from build123d import *

# Parameters (mm, degrees)
SKETCH1_W           = 67.8
SKETCH1_H           = 11.732307158
SKETCH1_R           = 1.25
BOSS_EXTRUDE1_DEPTH = 3
SKETCH1_7_R         = 0.5
BOSS_EXTRUDE2_DEPTH = 2
FILLET1_R           = 6


with BuildPart() as part:
    # Sketch1 → Boss-Extrude1 (new body)
    with BuildSketch(Plane(origin=(0, 0, 0), x_dir=(1, 0, 0), z_dir=(0, 1, 0))):
        with Locations((8.337190195, 0)):
            Rectangle(SKETCH1_W, SKETCH1_H)
        with Locations(Location((-4.662809805, -3.5, 0), (0, 0, 270))):
            Circle(SKETCH1_R, mode=Mode.SUBTRACT)
        with BuildLine():
            ThreePointArc((-15.948035413, -2.8), (-22.562809805, 0), (-15.948035413, 2.8))
            Line((-15.948035413, 2.8), (-3.54760873, 2.1))
            ThreePointArc((-3.54760873, 2.1), (-1.562809805, 0), (-3.54760873, -2.1))
            Line((-3.54760873, -2.1), (-15.948035413, -2.8))
        make_face(mode=Mode.SUBTRACT)
        with Locations(Location((-4.662809805, 3.5, 0), (0, 0, 270))):
            Circle(SKETCH1_R, mode=Mode.SUBTRACT)
        with BuildLine():
            Line((32.622415803, -2.8), (20.221989119, -2.1))
            ThreePointArc((20.221989119, -2.1), (18.237190195, 0), (20.221989119, 2.1))
            Line((20.221989119, 2.1), (32.622415803, 2.8))
            ThreePointArc((32.622415803, 2.8), (36.85745002, 3.591491343), (39.237190195, 0))
            ThreePointArc((39.237190195, 0), (36.85745002, -3.591491343), (32.622415803, -2.8))
        make_face(mode=Mode.SUBTRACT)
    extrude(amount=BOSS_EXTRUDE1_DEPTH)

    # Sketch1<7> → Boss-Extrude2 (add)
    # profile 1 of 2: a face of its own
    with BuildSketch(Plane(origin=(0, 0, 0), x_dir=(1, 0, 0), z_dir=(0, 1, 0))):
        with BuildLine():
            Line((-3.54760873, 2.1), (-15.948035413, 2.8))
            ThreePointArc((-15.948035413, 2.8), (-15.071318463, 1.520259825), (-14.762809805, 0))
            ThreePointArc((-14.762809805, 0), (-15.071318463, -1.520259825), (-15.948035413, -2.8))
            Line((-15.948035413, -2.8), (-3.54760873, -2.1))
            ThreePointArc((-3.54760873, -2.1), (-1.562809805, 0), (-3.54760873, 2.1))
        make_face()
        with Locations(Location((-13.331400804, 0, 0), (0, 0, 270))):
            Circle(SKETCH1_7_R, mode=Mode.SUBTRACT)
        with Locations(Location((-11.331400804, 0, 0), (0, 0, 270))):
            Circle(SKETCH1_7_R, mode=Mode.SUBTRACT)
        with Locations(Location((-9.331400804, 0, 0), (0, 0, 270))):
            Circle(SKETCH1_7_R, mode=Mode.SUBTRACT)
        with Locations(Location((-7.331400804, 0, 0), (0, 0, 270))):
            Circle(SKETCH1_7_R, mode=Mode.SUBTRACT)
        with Locations(Location((-5.331400804, 0, 0), (0, 0, 270))):
            Circle(SKETCH1_7_R, mode=Mode.SUBTRACT)
        with Locations(Location((-3.331400804, 0, 0), (0, 0, 270))):
            Circle(SKETCH1_7_R, mode=Mode.SUBTRACT)
    # profile 2 of 2: a face of its own
    with BuildSketch(Plane(origin=(0, 0, 0), x_dir=(1, 0, 0), z_dir=(0, 1, 0))):
        with BuildLine():
            ThreePointArc((20.221989119, 2.1), (18.237190195, 0), (20.221989119, -2.1))
            Line((20.221989119, -2.1), (32.622415803, -2.8))
            ThreePointArc((32.622415803, -2.8), (31.437190195, 0), (32.622415803, 2.8))
            Line((32.622415803, 2.8), (20.221989119, 2.1))
        make_face()
        with Locations(Location((22.005781193, 0, 0), (0, 0, 270))):
            Circle(SKETCH1_7_R, mode=Mode.SUBTRACT)
        with Locations(Location((24.005781193, 0, 0), (0, 0, 270))):
            Circle(SKETCH1_7_R, mode=Mode.SUBTRACT)
        with Locations(Location((26.005781193, 0, 0), (0, 0, 270))):
            Circle(SKETCH1_7_R, mode=Mode.SUBTRACT)
        with Locations(Location((28.005781193, 0, 0), (0, 0, 270))):
            Circle(SKETCH1_7_R, mode=Mode.SUBTRACT)
        with Locations(Location((30.005781193, 0, 0), (0, 0, 270))):
            Circle(SKETCH1_7_R, mode=Mode.SUBTRACT)
        with Locations(Location((20.005781193, 0, 0), (0, 0, 270))):
            Circle(SKETCH1_7_R, mode=Mode.SUBTRACT)
    extrude(amount=BOSS_EXTRUDE2_DEPTH)

    # Fillet1
    # the kernel refuses this fillet: 6 mm, written as the material it takes off along each edge
    with BuildSketch(Plane(origin=(-25.562809805, -15, 5.866153579), x_dir=(1, 0, 0), z_dir=(0, 1, 0)), Plane(origin=(42.237190195, -15, -5.866153579), x_dir=(-1, 0, 0), z_dir=(0, 1, 0))) as fillet1_piece_1:
        with BuildLine():
            CenterArc((FILLET1_R, FILLET1_R), FILLET1_R, 180, 90)
            Line((0, FILLET1_R), (0, 0))
            Line((0, 0), (FILLET1_R, 0))
        make_face()
    extrude(amount=33, mode=Mode.SUBTRACT)
    with BuildSketch(Plane(origin=(-25.562809805, -15, -5.866153579), x_dir=(1, 0, 0), z_dir=(0, 1, 0)), Plane(origin=(42.237190195, -15, 5.866153579), x_dir=(-1, 0, 0), z_dir=(0, 1, 0))) as fillet1_piece_2:
        with BuildLine():
            CenterArc((FILLET1_R, -FILLET1_R), FILLET1_R, 90, 90)
            Line((0, -FILLET1_R), (0, 0))
            Line((0, 0), (FILLET1_R, 0))
        make_face()
    extrude(amount=33, mode=Mode.SUBTRACT)


solid = part.part
Check sheet for the modelled part. Datum: model origin and axes. Units: mm. A direction names the side the tool comes from. Round coordinates to 2 decimals unless told otherwise and drop trailing zeros. Loops run counter-clockwise (first coordinate to the right, second up) from the corner with the lowest first, then second, coordinate; pieces in that order, holes last.
1. Mould release check, pull along X, two halves, no side actions. Record for faces 3 (the cylindrical face through (-23.71, 1.48, -4.2)), 4 (the cylindrical face through (-5.77, 1.48, -2.92)), 5 (the flat face through (8, 3, 0)): released by +X, released by -X, zero draft, split by the parting line, or undercut.
2. Set-up check for faces 1 (the cylindrical face through (-1.563, 2.493, -0.045)), 2 (the cylindrical face through (-5.77, 1.48, 4.08)): record each of +Z, -Z, +X, -X, +Y, -Y from which the full face is reachable in a straight line by a thin tool's end or side.
3. Sectioned sample at B-B on y = 1.1. Give the number of separate pieces and of enclosed holes in the cut face, and give its area (3 significant figures).
4. Gauge pin test, flat end, axial feed: pin 1 Ø7 at (x, z) = (-18.66, 0) entering from +Y. Record the tip position at first contact, or that the pin passes through.
5. Sectioned sample at A-A on x = -20.5. Record the boundary of the cut face in (y, z), and give its area (3 significant figures).
6. Sectioned sample at D-D on x = 37.5. Record the boundary of the cut face in (y, z), and give its area (3 significant figures).
7. Sectioned sample at C-C on z = 1.5. Record the boundary of the cut face in (x, y).
8. Scan lines: probe 1 along X at (y, z) = (1.25, 1.5); probe 2 along Z at (x, y) = (24, 0.25); probe 3 along X at (y, z) = (0.3, -1). Record each from-to range of solid material in increasing order.
Recorded:
1. face 3: released by -X
1. face 4: undercut
1. face 5: zero draft
2. face 1: +Y
2. face 2: +Y, -Y
3. separate pieces: 1
3. enclosed holes: 16
3. area: 650 mm2
4. pin 1: passes through
5. outline: (0, -5.79) - (3, -5.79) - (3, -3.44) - (0, -3.44) - close; (0, 3.44) - (3, 3.44) - (3, 5.79) - (0, 5.79) - close
5. area: 14.1 mm2
6. outline: (0, -5.73) - (3, -5.73) - (3, -3.25) - (0, -3.25) - close; (0, 3.25) - (3, 3.25) - (3, 5.73) - (0, 5.73) - close
6. area: 14.9 mm2
7. outline: (-25.34, 0) - (-22.26, 0) - (-22.26, 3) - (-25.34, 3) - close; (-15.06, 0) - (31.74, 0) - (31.74, 2) - (18.87, 2) - (18.87, 3) - (-2.19, 3) - (-2.19, 2) - (-15.06, 2) - close; (38.94, 0) - (42.01, 0) - (42.01, 3) - (38.94, 3) - close
8. probe 1: x = -25.34 to -22.26, -15.06 to 31.74, 38.94 to 42.01
8. probe 2: z = -5.87 to -0.5, 0.5 to 5.87
8. probe 3: x = -25.45 to -22.43, -14.89 to 31.57, 39.11 to 42.13
